from build123d import *

# Parameters (mm, degrees)
F0_W            = 762
F0_H            = 146.05
F1_DEPTH        = 31.75
F2_R            = 9.525
F3_DEPTH        = 762.001
F4_R            = 9.525
F5_DEPTH        = 146.051
F6_R            = 9.525
F7_DEPTH        = 762.0010001
F8_R            = 9.5195259248
F9_DEPTH        = 146.0510001
F11_D           = 12.7
F11_DEPTH       = 19.05
F11_TIP         = 3.8154649308
F12_D           = 5.5
F12_CSINK_D     = 11.2
F12_CSINK_ANGLE = 90
F14_D           = 5.1054
F14_CSINK_D     = 10.4394
F14_CSINK_ANGLE = 82


with BuildPart() as f1:
    # F0 (on Front) → F1 (new body)
    with BuildSketch(Plane.XZ):
        Rectangle(F0_W, F0_H)
    extrude(amount=F1_DEPTH)

    # F2 (on face) → F3 (cut, through all)
    with BuildSketch(Plane(origin=(-381, 0, 0), x_dir=(0, -1, 0), z_dir=(-1, 0, 0))):
        with Locations((31.75, 73.025)):
            Circle(F2_R)
    extrude(amount=-F3_DEPTH, mode=Mode.SUBTRACT)

    # F4 (on face) → F5 (cut, through all)
    with BuildSketch(Plane.XY.offset(73.025)):
        with Locations((-380.995452404, -31.7343771458)):
            Circle(F4_R)
    extrude(amount=-F5_DEPTH, mode=Mode.SUBTRACT)

    # F6 (on face) → F7 (cut, through all)
    with BuildSketch(Plane.YZ.offset(381)):
        with Locations((-31.75, -73.025)):
            Circle(F6_R)
    extrude(amount=-F7_DEPTH, mode=Mode.SUBTRACT)

    # F8 (on face) → F9 (cut, through all)
    with BuildSketch(Plane(origin=(0, 0, -73.025), x_dir=(1, 0, 0), z_dir=(0, 0, -1))):
        with Locations((381.0260295868, 31.7688845098)):
            Circle(F8_R)
    extrude(amount=-F9_DEPTH, mode=Mode.SUBTRACT)

    # F11
    with Locations(Plane.XZ.offset(31.75)):
        with Locations((-304.7976701619, 0.8426916512), (-152.3976701619, 0.8426916512), (0.466863421, 0.8401229861), (152.866863421, 0.8401229861), (305.266863421, 0.8401229861)):
            Hole(F11_D / 2, depth=F11_DEPTH)
            with Locations((0, 0, -(F11_DEPTH + F11_TIP / 2))):  # 118° drill point
                Cone(0, F11_D / 2, F11_TIP, mode=Mode.SUBTRACT)

    # F12 (through all)
    with Locations(Plane(origin=(0, 0, 0), x_dir=(1, 0, 0), z_dir=(0, 1, 0))):
        with Locations((304.8, 0), (152.4, 0), (0, 0), (-152.4, 0), (-304.8, 0)):
            CounterSinkHole(F12_D / 2, F12_CSINK_D / 2, counter_sink_angle=F12_CSINK_ANGLE)

    # F14 (through all)
    with Locations(Plane.XZ.offset(31.75)):
        with Locations((-203.2, 0), (203.2, 0)):
            CounterSinkHole(F14_D / 2, F14_CSINK_D / 2, counter_sink_angle=F14_CSINK_ANGLE)


solid = f1.part
Source: CAD feature listing. Evaluate the final solid. Frame: model axes, mm. A direction names the side the tool comes from. Give positions to 0.01 mm unless a question says otherwise; leave off trailing zeros. Write each loop counter-clockwise with the first axis right and the second up, starting at its lowest first coordinate (ties: lowest second). Pieces come first, ordered by that corner, then holes. Notation, with made-up numbers: M 85,77 L 101,77 A20 cw 101,85 Z; hole C 58,30.5 d1. An arc over 180 degrees is marked long. Answer as a JSON object with one key per item and string values.
Q1. Contact query for flat-ended pins moving along their axis: P1, Ø10, axis at x = 152.87, z = 0.84, coming from the -Y side; P2, Ø5, axis at x = 304.8, z = 0, coming from the -Y side; P3, Ø9, axis at x = 0, z = 0, coming from the -Y side; P4, Ø6.5, axis at x = -304.8, z = 0, coming from the +Y side. Output: stop coordinate, or through.
Geometry check:
{"P1": "stops at y = -11.89", "P2": "passes through", "P3": "stops at y = -12.17", "P4": "stops at y = -2.35"}
Q2. Mould query, pull axis Z, two halves, no side actions, for faces 1 (the face through (-5, -11, 73.025)), 2 (the face through (-381, -11, -1)), 3 (the face through (-5, -11, -73.025)), 4 (the face through (1.58, -10.13, 2.59)). Classes: +Z half, -Z half, draft (parallel to the pull), parting line (faces both ways), or undercut.
Geometry check:
{"face 1": "+Z half", "face 2": "draft", "face 3": "-Z half", "face 4": "undercut"}
Q3. Access query for faces 5 (the face through (-5.59, -22.09, 2.75)), 6 (the face through (-5, 0, 17)). Directions: +Z, -Z, +X, -X, +Y, -Y. A direction counts if a zero-diameter tool reaches every point of the face in a straight line with its end or side. Return the directions, or none.
Geometry check:
{"face 5": "-Y", "face 6": "+Z, -Z, +X, -X, +Y"}
Q4. Cut plane A-A, the plane x = -180.5. Return the cut outline in (y, z) (3 decimals), then the cut area to 3 significant figures.
Geometry check:
{"outline": "M -31.75,-63.5 A9.525 cw -22.225,-73.025 L 0,-73.025 L 0,73.025 L -22.225,73.025 A9.525 cw -31.75,63.5 Z", "area": "4,490 mm^2"}
Q5. Ray query, line 1 along Z through (x, y) = (152.4, -8) (3 decimals); line 2 along Z through (x, y) = (304, -25); line 3 along X through (y, z) = (-25.5, -38). Return the intervals inside material, ascending.
Geometry check:
{"line 1": "z = -73.025 to -2.75, 2.75 to 73.025", "line 2": "z = -66.3 to -5.38, 7.06 to 66.3", "line 3": "x = -373.79 to 373.86"}
